Could you check a few things on this model? Use its own coordinates, in mm. Round coordinates to 2 decimals unless told otherwise and drop trailing zeros. Loops run counter-clockwise (first coordinate to the right, second up) from the corner with the lowest first, then second, coordinate; pieces in that order, holes last. Notation, with made-up numbers: (66, 58) -> (77, 58) arc R23 ccw to (77, 66) -> close; hole circle Ø9 at (-5.75, -27.75). An arc over 180 degrees is marked (long way). One line per item, written item: value.
```python
from build123d import *

# Parameters (mm, degrees)
SKETCH_1_R          = 3
EXTRUDE_1_DEPTH     = 2
SKETCH_2_W          = 15
SKETCH_2_H          = 129
CUT_EXTRUDE_1_DEPTH = 174.643312569
SKETCH_3_W          = 40
SKETCH_3_H          = 74
CUT_EXTRUDE_2_DEPTH = 174.643312569
SKETCH_4_W          = 70
SKETCH_4_H          = 20
SKETCH_4_W_2        = 25
SKETCH_4_H_2        = 70
CUT_EXTRUDE_3_DEPTH = 174.643312569


with BuildPart() as part:
    # Эскиз1 → Бобышка-Вытянуть1 (new body)
    with BuildSketch(Plane(origin=(0, 0, 0), x_dir=(1, 0, 0), z_dir=(0, 1, 0))):
        Polygon((-143, 72), (158, 72), (158, -72), (-143, -72), (-158, -72), (-158, 72), align=None)
        with Locations(Location((-138.5, 67.5, 0), (0, 0, 270))):
            Circle(SKETCH_1_R, mode=Mode.SUBTRACT)
        with Locations(Location((-150.5, -64.5, 0), (0, 0, 270))):
            Circle(SKETCH_1_R, mode=Mode.SUBTRACT)
        with Locations(Location((150.5, -64.5, 0), (0, 0, 270))):
            Circle(SKETCH_1_R, mode=Mode.SUBTRACT)
        with Locations(Location((138.5, 67.5, 0), (0, 0, 270))):
            Circle(SKETCH_1_R, mode=Mode.SUBTRACT)
    extrude(amount=EXTRUDE_1_DEPTH)

    # Эскиз2 → Вырез-Вытянуть1 (cut, through all)
    with BuildSketch(Plane(origin=(0, 2, 0), x_dir=(1, 0, 0), z_dir=(0, 1, 0))):
        with Locations((150.5, 7.5)):
            Rectangle(SKETCH_2_W, SKETCH_2_H)
        with Locations((-150.5, 7.5)):
            Rectangle(SKETCH_2_W, SKETCH_2_H)
    extrude(amount=-CUT_EXTRUDE_1_DEPTH, mode=Mode.SUBTRACT)

    # Эскиз3 → Вырез-Вытянуть2 (cut, through all)
    with BuildSketch(Plane(origin=(0, 2, 0), x_dir=(1, 0, 0), z_dir=(0, 1, 0))):
        with Locations((0, -35)):
            Rectangle(SKETCH_3_W, SKETCH_3_H)
    extrude(amount=-CUT_EXTRUDE_2_DEPTH, mode=Mode.SUBTRACT)

    # Эскиз4 → Вырез-Вытянуть3 (cut, through all)
    with BuildSketch(Plane(origin=(0, 2, 0), x_dir=(1, 0, 0), z_dir=(0, 1, 0))):
        with Locations((-88, 47)):
            Rectangle(SKETCH_4_W, SKETCH_4_H)
        with Locations((-110.5, -13)):
            Rectangle(SKETCH_4_W_2, SKETCH_4_H_2)
        with Locations((-65.5, -13)):
            Rectangle(SKETCH_4_W_2, SKETCH_4_H_2)
        with Locations((65.5, -13)):
            Rectangle(SKETCH_4_W_2, SKETCH_4_H_2)
        with Locations((110.5, -13)):
            Rectangle(SKETCH_4_W_2, SKETCH_4_H_2)
        with Locations((88, 47)):
            Rectangle(SKETCH_4_W, SKETCH_4_H)
    extrude(amount=-CUT_EXTRUDE_3_DEPTH, mode=Mode.SUBTRACT)


solid = part.part
```
(1) For pin 1 Ø1 at (y, z) = (1, -3.5) entering from -X; pin 2 Ø0.6 at (y, z) = (0.5, -27.5) entering from +X; pin 3 Ø1 at (x, y) = (-1.5, 1.5) entering from +Z, each with a flat end and sliding along its axis, tell me the tip position at first contact or that it passes through.
Results below:
pin 1: stops at x = -143
pin 2: stops at x = 143
pin 3: stops at z = -2
(2) Imagine slicing it at D-D on z = 64.5. Write out the boundary of the cut face in (x, y).
Results below:
outline: (-158, 0) -> (-153.5, 0) -> (-153.5, 2) -> (-158, 2) -> close; (-147.5, 0) -> (-20, 0) -> (-20, 2) -> (-147.5, 2) -> close; (20, 0) -> (147.5, 0) -> (147.5, 2) -> (20, 2) -> close; (153.5, 0) -> (158, 0) -> (158, 2) -> (153.5, 2) -> close
(3) Please list where these lines run through material, in increasing order: L1, parallel to Z at x = -118, y = 0.1; L2, parallel to X at y = 1.15, z = 64.5; L3, parallel to X at y = 0.7, z = -54.
Results below:
L1: z = -72 to -57, -37 to -22, 48 to 72
L2: x = -158 to -153.5, -147.5 to -20, 20 to 147.5, 153.5 to 158
L3: x = -143 to -123, -53 to 53, 123 to 143
(4) Imagine slicing it at B-B on x = -106. Write out the boundary of the cut face in (y, z).
Results below:
outline: (0, -72) -> (2, -72) -> (2, -57) -> (0, -57) -> close; (0, -37) -> (2, -37) -> (2, -22) -> (0, -22) -> close; (0, 48) -> (2, 48) -> (2, 72) -> (0, 72) -> close
(5) We'd pull the mould along X, two halves only. Please class faces 1 (the face through (-147.526, 0.986, 64.109)), 2 (the face through (2, 2, -17)): +X half, -X half, draft (parallel to the pull), parting line (faces both ways), or undercut.
Results below:
face 1: undercut
face 2: draft
(6) Imagine slicing it at A-A on x = -138.5. Write out the boundary of the cut face in (y, z).
Results below:
outline: (0, -72) -> (2, -72) -> (2, -70.5) -> (0, -70.5) -> close; (0, -64.5) -> (2, -64.5) -> (2, 72) -> (0, 72) -> close
(7) Imagine slicing it at C-C on z = 31. Write out the boundary of the cut face in (x, y).
Results below:
outline: (-143, 0) -> (-123, 0) -> (-123, 2) -> (-143, 2) -> close; (-98, 0) -> (-78, 0) -> (-78, 2) -> (-98, 2) -> close; (-53, 0) -> (-20, 0) -> (-20, 2) -> (-53, 2) -> close; (20, 0) -> (53, 0) -> (53, 2) -> (20, 2) -> close; (78, 0) -> (98, 0) -> (98, 2) -> (78, 2) -> close; (123, 0) -> (143, 0) -> (143, 2) -> (123, 2) -> close
